```python
from build123d import *

# Parameters (mm, degrees)
SKETCH2_R           = 50
SKETCH2_R_2         = 5
BOSS_EXTRUDE1_DEPTH = 100
BOSS_EXTRUDE2_DEPTH = 10
SKETCH4_W           = 25
SKETCH4_H           = 30
BOSS_EXTRUDE3_DEPTH = 100
SKETCH5_R           = 10
BOSS_EXTRUDE4_DEPTH = 50


with BuildPart() as part:
    # Sketch2 → Boss-Extrude1 (new body)
    with BuildSketch(Plane(origin=(0, 0, 0), x_dir=(1, 0, 0), z_dir=(0, 1, 0))):
        with Locations(Location((0, 0, 0), (0, 0, 270))):
            Circle(SKETCH2_R)
        with Locations(Location((0, 0, 0), (0, 0, 270))):
            Circle(SKETCH2_R_2, mode=Mode.SUBTRACT)
    extrude(amount=BOSS_EXTRUDE1_DEPTH)

    # Sketch3 → Boss-Extrude2 (add)
    with BuildSketch(Plane.XZ):
        with BuildLine():
            Line((-47.696960071, -15), (-100, -15))
            Line((-100, -15), (-100, 15))
            Line((-100, 15), (-47.696960071, 15))
            ThreePointArc((-47.696960071, 15), (-50, 0), (-47.696960071, -15))
        make_face()
    extrude(amount=-BOSS_EXTRUDE2_DEPTH)

    # Sketch4 → Boss-Extrude3 (add)
    with BuildSketch(Plane.XZ):
        with Locations((-100, 0)):
            Rectangle(SKETCH4_W, SKETCH4_H)
    extrude(amount=-BOSS_EXTRUDE3_DEPTH)

    # Sketch5 → Boss-Extrude4 (add)
    with BuildSketch(Plane.ZY.offset(112.5)):
        with Locations((0, 50)):
            Circle(SKETCH5_R)
    extrude(amount=BOSS_EXTRUDE4_DEPTH)


solid = part.part
```
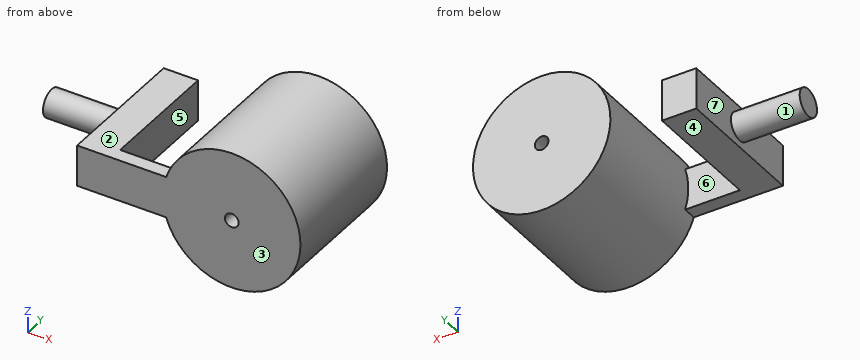
Geometry check sheet. Reference: the model listing, model coordinates, mm. Face numbers are marked on the shaded views. A direction names the side the tool comes from. Round coordinates to 2 decimals unless told otherwise and drop trailing zeros. Order: outer loops, then holes, each group sorted by start corner. A loop starts at its lowest first (then second) coordinate and runs counter-clockwise, first axis right, second up. Notation, with made-up numbers: (1, 80.25) - (37, 80.25) arc R19 cw to (37, 86.25) - close; hole circle Ø4 at (35, 32). An arc over 180 degrees is marked (long way). Use a Markdown table: item, result. Add a question column.
1) Mould release check, pull along X, two halves, no side actions. Record for the marked faces 4, 5, 6 and 7: released by +X, released by -X, zero draft, split by the parting line, or undercut.
2) Set-up check for the marked faces 1, 2 and 3: record each of +Z, -Z, +X, -X, +Y, -Y from which the full face is reachable in a straight line by a thin tool's end or side.
3) Section check C-C (z = 0). Record the cut outline in (x, y).
4) Gauge pin test, flat ends, axial feed: P1, Ø8, axis at y = 11.5, z = -7.5, coming from the +X side; P2, Ø9, axis at x = 0, z = 0, coming from the +Y side; P3, Ø5, axis at x = 5, y = 32, coming from the -Z side; P4, Ø9, axis at x = -67, z = -2.5, coming from the +Y side. Record the tip position at first contact, or that the pin passes through.
5) Section check A-A (y = 50). Record the cut outline in (x, z), then the cut area to 3 significant figures.
6) Section check D-D (y = 18). Record the cut outline in (x, z), then the cut area to 3 significant figures.
7) Thickness scan on line 1 along X through (y, z) = (56, 0); line 2 along X through (y, z) = (34, 0); line 3 along X through (y, z) = (40, 12). Record the ranges inside material, lowest first.
8) Section check B-B (x = 0). Record the cut outline in (y, z), then the cut area to 3 significant figures.
Established:
| question | item | result |
|---|---|---|
| 1 | face 4 | zero draft |
| 1 | face 5 | undercut |
| 1 | face 6 | undercut |
| 1 | face 7 | released by -X |
| 2 | face 1 | -X |
| 2 | face 2 | +Z, -X, +Y, -Y |
| 2 | face 3 | +Z, -Z, +X, -X, -Y |
| 3 | outline | (-162.5, 40) - (-112.5, 40) - (-112.5, 0) - (-5, 0) - (-5, 100) - (-50, 100) - (-50, 10) - (-87.5, 10) - (-87.5, 100) - (-112.5, 100) - (-112.5, 60) - (-162.5, 60) - close; (5, 0) - (50, 0) - (50, 100) - (5, 100) - close |
| 4 | P1 | x = 49.88 |
| 4 | P2 | through |
| 4 | P3 | z = -49.94 |
| 4 | P4 | y = 10 |
| 5 | outline | (-162.5, -10) - (-112.5, -10) - (-112.5, -15) - (-87.5, -15) - (-87.5, 15) - (-112.5, 15) - (-112.5, 10) - (-162.5, 10) - close; circle Ø100 at (0, 0); hole circle Ø10 at (0, 0) |
| 5 | area | 9,530 mm2 |
| 6 | outline | (-112.5, -15) - (-87.5, -15) - (-87.5, 15) - (-112.5, 15) - close; circle Ø100 at (0, 0); hole circle Ø10 at (0, 0) |
| 6 | area | 8,530 mm2 |
| 7 | line 1 | -162.5 to -87.5, -50 to -5, 5 to 50 |
| 7 | line 2 | -112.5 to -87.5, -50 to -5, 5 to 50 |
| 7 | line 3 | -112.5 to -87.5, -48.54 to 48.54 |
| 8 | outline | (0, -50) - (100, -50) - (100, -5) - (0, -5) - close; (0, 5) - (100, 5) - (100, 50) - (0, 50) - close |
| 8 | area | 9,000 mm2 |
